Can you work these out from the model? Positions are in its coordinate system, mm. A direction names the side the tool comes from. Give positions to 0.01 mm unless a question says otherwise; leave off trailing zeros. Order: outer loops, then holes, each group sorted by start corner. A loop starts at its lowest first (then second) coordinate and runs counter-clockwise, first axis right, second up. Notation, with made-up numbers: (49, 52) -> (76, 52) arc R22 ccw to (76, 59) -> close; hole circle Ø9 at (39, -17.75). An arc over 180 degrees is marked (long way). Answer as CSV lines item,"result".
```python
from build123d import *

# Parameters (mm, degrees)
EXTRUDE_1_DEPTH      = 4
SKETCH_3_W           = 15.588457268
SKETCH_3_H           = 4
EXTRUDE_3_DEPTH      = 2
SKETCH_19_W          = 15.588457268
SKETCH_19_H          = 4
EXTRUDE_5_DEPTH      = 5
SKETCH_4_W           = 5
SKETCH_4_H           = 4
EXTRUDE_6_DEPTH      = 5
SKETCH_22_R          = 2
CUT_EXTRUDE_17_DEPTH = 150
CHAMFER_1_SIZE       = 3
EXTRUDE_7_DEPTH      = 4
SKETCH_27_W          = 5
SKETCH_27_H          = 4
SKETCH_27_W_2        = 6.299038106
CUT_EXTRUDE_19_DEPTH = 1
CUT_EXTRUDE_22_DEPTH = 5


with BuildPart() as part:
    # 草图1 → 凸台-拉伸1 (new body)
    with BuildSketch(Plane.XY):
        Polygon((-111.620742166, 100.372452405), (-127.209199434, 100.372452405), (-127.251564891, 105.942182287), (-111.620742166, 114.966641994), align=None)
    extrude(amount=EXTRUDE_1_DEPTH)

    # 草图3 → 凸台-拉伸3 (add)
    with BuildSketch(Plane.XZ.offset(-100.372452405)):
        with Locations((-119.4149708, 2)):
            Rectangle(SKETCH_3_W, SKETCH_3_H)
    extrude(amount=EXTRUDE_3_DEPTH)

    # 草图19 → 凸台-拉伸5 (add)
    with BuildSketch(Plane.XZ.offset(-98.372452405)):
        with Locations((-119.4149708, 2)):
            Rectangle(SKETCH_19_W, SKETCH_19_H)
    extrude(amount=EXTRUDE_5_DEPTH)

    # 草图4 → 凸台-拉伸6 (add)
    with BuildSketch(Plane(origin=(-77.687201819, 134.558180648, 0), x_dir=(0.8660254037844398, 0.49999999999999806, 0), z_dir=(-0.499999999999998, 0.8660254037844397, 0))):
        with Locations((-54.731996723, -2)):
            Rectangle(SKETCH_4_W, SKETCH_4_H)
        with Locations((-41.683077308, -2)):
            Rectangle(SKETCH_4_W, SKETCH_4_H)
    extrude(amount=EXTRUDE_6_DEPTH)

    # 草图22 → 切除-拉伸17 (cut)
    with BuildSketch(Plane(origin=(0.801824419, -4.558538123, 5), x_dir=(0.9999710727819138, 0.007606155361845765, 0), z_dir=(0, 0, 1))):
        with Locations(Location((-119.468439353, 102.928528754, 0), (0, 0, 179.564195197))):
            Circle(SKETCH_22_R)
    extrude(amount=-CUT_EXTRUDE_17_DEPTH, mode=Mode.SUBTRACT)

    # 倒角1
    chamfer_1_edges = [part.edges().sort_by_distance(p)[0] for p in [
        (-127.209199434, 93.372452405, 2),
        (-111.620742166, 93.372452405, 2),
    ]]
    chamfer(chamfer_1_edges, length=CHAMFER_1_SIZE)

    # 草图25 → 凸台-拉伸7 (add)
    with BuildSketch(Plane(origin=(0, 0, 0), x_dir=(-1, 0, 0), z_dir=(0, 0, -1))):
        Polygon((111.620742166, 96.372452405), (111.620742166, 114.966641994), (114.120742166, 119.296769013), (112.995742166, 119.946288066), (110.120742166, 114.966641994), (110.120742166, 97.872452405), align=None)
    extrude(amount=-EXTRUDE_7_DEPTH)

    # 草图27 → 切除-拉伸19 (cut)
    with BuildSketch(Plane(origin=(-80.187201819, 138.888307667, 0), x_dir=(0.8660254037844395, 0.4999999999999986, 0), z_dir=(-0.4999999999999986, 0.8660254037844395, 0))):
        with Locations((-54.731996723, -2)):
            Rectangle(SKETCH_27_W, SKETCH_27_H)
        with Locations((-41.033558255, -2)):
            Rectangle(SKETCH_27_W_2, SKETCH_27_H)
    extrude(amount=-CUT_EXTRUDE_19_DEPTH, mode=Mode.SUBTRACT)

    # 草图30 → 切除-拉伸22 (cut)
    with BuildSketch(Plane(origin=(0.801824419, -4.558538123, 0), x_dir=(-0.9999710727819139, -0.007606155361845766, 0), z_dir=(0, 0, -1))):
        with BuildLine():
            Line((116.661773389, 114.005519488), (117.895269421, 116.180028062))
            Line((117.895269421, 116.180028062), (118.865299077, 117.929039916))
            Line((118.865299077, 117.929039916), (121.330841562, 116.561611031))
            Line((121.330841562, 116.561611031), (120.330719024, 114.798512507))
            Line((120.330719024, 114.798512507), (119.097222993, 112.624003932))
            Line((119.097222993, 112.624003932), (120.010516594, 112.105935599))
            ThreePointArc((120.010516594, 112.105935599), (120.15167585, 111.924842132), (120.123438099, 111.696975046))
            Line((120.123438099, 111.696975046), (119.185981115, 110.04434853))
            ThreePointArc((119.185981115, 110.04434853), (119.004887648, 109.903189273), (118.777020562, 109.931427025))
            Line((118.777020562, 109.931427025), (117.82023679, 110.474165279))
            Line((117.82023679, 110.474165279), (117.721557107, 110.300204593))
            ThreePointArc((117.721557107, 110.300204593), (117.54046364, 110.159045336), (117.312596554, 110.187283087))
            Line((117.312596554, 110.187283087), (115.486009352, 111.223419754))
            ThreePointArc((115.486009352, 111.223419754), (115.344850096, 111.404513221), (115.373087847, 111.632380307))
            Line((115.373087847, 111.632380307), (115.471767529, 111.806340993))
            Line((115.471767529, 111.806340993), (114.514983756, 112.349079246))
            ThreePointArc((114.514983756, 112.349079246), (114.3738245, 112.530172713), (114.402062251, 112.758039799))
            Line((114.402062251, 112.758039799), (115.339519235, 114.410666316))
            ThreePointArc((115.339519235, 114.410666316), (115.520612702, 114.551825572), (115.748479788, 114.523587821))
            Line((115.748479788, 114.523587821), (116.661773389, 114.005519488))
        make_face()
    extrude(amount=-CUT_EXTRUDE_22_DEPTH, mode=Mode.SUBTRACT)


solid = part.part
```
Item 1: For pin 1 (2 mm diameter, centred on x = -125.5, z = 1.5, fed in from -Y); pin 2 (2 mm diameter, centred on y = 98.5, z = 2, fed in from -X), each with a flat end and sliding along its axis, tell me the tip position at first contact or that it passes through.
Numbers:
pin 1,"stops at y = 93.66"
pin 2,"stops at x = -127.21"
Item 2: Imagine slicing it at D-D, the plane x = -121.75. Please give me the cut outline in (y, z).
Numbers:
outline,"(93.37, 0) -> (109.12, 0) -> (109.12, 4) -> (93.37, 4) -> close"
Item 3: For faces 1 (the flat face through (-118.338, 104.737, 1.972)), 2 (the flat face through (-119, 93.372, 2)), 3 (the flat face through (-123.907, 110.15, 2.028)), which set-ups out of +Z, -Z, +X, -X, +Y, -Y let a thin tool reach every point of the face, with its end or its side?
Numbers:
face 1,"+Z, -Z"
face 2,"+Z, -Z, +X, -X, -Y"
face 3,"+Z, -Z, +Y"
Item 4: Imagine slicing it at A-A, the plane y = 99. Please give me the cut outline in (x, z), then the cut area to 3 significant figures.
Numbers:
outline,"(-127.21, 0) -> (-120.72, 0) -> (-120.72, 4) -> (-127.21, 4) -> close; (-118.17, 0) -> (-110.12, 0) -> (-110.12, 4) -> (-118.17, 4) -> close"
area,"58.2 mm²"
Item 5: We'd pull the mould along Y, two halves only. Please class faces 4 (the flat face through (-117, 104, 4)), 5 (the flat face through (-127.117, 110.639, 1.972)), 6 (the flat face through (-114.9, 108.1, 2)): released by +Y, released by -Y, zero draft, split by the parting line, or undercut.
Numbers:
face 4,"zero draft"
face 5,"released by +Y"
face 6,"undercut"
Item 6: Imagine slicing it at B-B, the plane x = -116.25. Please give me the cut outline in (y, z).
Numbers:
outline,"(93.37, 0) -> (105.37, 0) -> (105.37, 4) -> (93.37, 4) -> close; (108.83, 0) -> (112.29, 0) -> (112.29, 4) -> (108.83, 4) -> close; (112.98, 0) -> (116.91, 0) -> (116.91, 4) -> (112.98, 4) -> close"
Item 7: Please list where these lines run through material, in increasing order: line 1 along Y through (x, z) = (-117, 2.05); line 2 along Y through (x, z) = (-118, 1.2); line 3 along X through (y, z) = (105.75, 3).
Numbers:
line 1,"y = 93.37 to 104.93, 109.03 to 111.86, 114.28 to 116.48"
line 2,"y = 93.37 to 96.08, 98.84 to 104.93, 110.77 to 111.28"
line 3,"x = -127.25 to -119.9, -115.58 to -110.12"
